For this review, take the finished solid that the model builds, in its own axes (mm). A direction names the side the tool comes from. Round coordinates to 2 decimals unless told otherwise and drop trailing zeros. Write each loop counter-clockwise with the first axis right and the second up, starting at its lowest first coordinate (ties: lowest second). Pieces come first, ordered by that corner, then holes. Notation, with made-up numbers: (10, 10) -> (63, 10) arc R19 cw to (63, 19) -> close; hole circle Ø1 at (-15, 35.5). An arc over 180 degrees is marked (long way). Answer in a Markdown table with one row per item.
from build123d import *

# Parameters (mm, degrees)
SKETCH1_R                       = 13.75
BOSS_EXTRUDE1_DEPTH             = 60
SKETCH5_R                       = 10.75
BOSS_EXTRUDE2_DEPTH             = 14.9
CUT_EXTRUDE1_START              = -20
CUT_EXTRUDE1_DEPTH              = 20
CUT_EXTRUDE2_DEPTH              = 64.072379058
CUT_EXTRUDE2_DEPTH_BACK         = 64.072379058
SKETCH7_R                       = 2.625
BOSS_EXTRUDE3_REACH             = 65.072
SKETCH8_R                       = 2.625
BOSS_EXTRUDE3_DIRECTION_2_REACH = 65.072
SKETCH9_R                       = 12.75
SKETCH9_R_2                     = 2.5
CUT_EXTRUDE3_DEPTH              = 10


with BuildPart() as part:
    # Sketch1 → Boss-Extrude1 (new body)
    with BuildSketch(Plane(origin=(0, 0, 0), x_dir=(1, 0, 0), z_dir=(0, 1, 0))):
        with Locations(Location((0, 0, 0), (0, 0, 270))):
            Circle(SKETCH1_R)
    extrude(amount=BOSS_EXTRUDE1_DEPTH)

    # Sketch5 → Boss-Extrude2 (add)
    with BuildSketch(Plane.XZ):
        with Locations(Location((0, 0, 0), (0, 0, 90))):
            Circle(SKETCH5_R)
        with BuildLine():
            Line((0.75, -9.219544457), (0.75, 9.219544457))
            ThreePointArc((0.75, 9.219544457), (9.25, 0), (0.75, -9.219544457))
        make_face(mode=Mode.SUBTRACT)
        with BuildLine():
            Line((-0.75, 9.219544457), (-0.75, -9.219544457))
            ThreePointArc((-0.75, -9.219544457), (-9.25, 0), (-0.75, 9.219544457))
        make_face(mode=Mode.SUBTRACT)
    extrude(amount=BOSS_EXTRUDE2_DEPTH)

    # Sketch6 → Cut-Extrude1 (cut)
    with BuildSketch(Plane.XZ.offset(CUT_EXTRUDE1_START)):
        with BuildLine():
            Line((-0.75, -9.219544457), (-0.75, 9.219544457))
            ThreePointArc((-0.75, 9.219544457), (-9.25, 0), (-0.75, -9.219544457))
        make_face()
        with BuildLine():
            ThreePointArc((0.75, -9.219544457), (9.25, 0), (0.75, 9.219544457))
            Line((0.75, 9.219544457), (0.75, -9.219544457))
        make_face()
    extrude(amount=CUT_EXTRUDE1_DEPTH, mode=Mode.SUBTRACT)

    # Sketch7 → Cut-Extrude2 (cut, two sides: drawn at the far end of the back side and taken through both)
    with BuildSketch(Plane(origin=(0, 0, 0), x_dir=(0, 0, -1), z_dir=(1, 0, 0)).offset(-CUT_EXTRUDE2_DEPTH_BACK)):
        with Locations((0, -10)):
            Circle(SKETCH7_R)
    extrude(amount=CUT_EXTRUDE2_DEPTH + CUT_EXTRUDE2_DEPTH_BACK, mode=Mode.SUBTRACT)

    # Boss-Extrude3: up to this face of the body (flat: up to its plane)
    boss_extrude3_end = Plane(part.part.faces().sort_by_distance((0.75, 2.986865704, 0))[0])
    # Sketch8 → Boss-Extrude3 (add, up to the picked face)
    with BuildSketch(Plane(origin=(0, 0, 0), x_dir=(0, 0, -1), z_dir=(1, 0, 0)), mode=Mode.PRIVATE) as boss_extrude3_sk1:
        with Locations((0, -10)):
            Circle(SKETCH8_R)
    boss_extrude3_tool1 = split(extrude(boss_extrude3_sk1.sketch, amount=BOSS_EXTRUDE3_REACH, mode=Mode.PRIVATE), bisect_by=boss_extrude3_end, keep=Keep.BOTH, mode=Mode.PRIVATE)
    add(boss_extrude3_tool1.solids().sort_by(Axis((0, -10, 0), (1, 0, 0)))[0])

    # Boss-Extrude3 direction 2: up to this face of the body (flat: up to its plane)
    boss_extrude3_direction_2_end = Plane(part.part.faces().sort_by_distance((-0.75, 2.986865704, 0))[0])
    # Sketch8 → Boss-Extrude3 direction 2 (add, up to the picked face)
    with BuildSketch(Plane(origin=(0, 0, 0), x_dir=(0, 0, -1), z_dir=(1, 0, 0)), mode=Mode.PRIVATE) as boss_extrude3_direction_2_sk1:
        with Locations((0, -10)):
            Circle(SKETCH8_R)
    boss_extrude3_direction_2_tool1 = split(extrude(boss_extrude3_direction_2_sk1.sketch, amount=-BOSS_EXTRUDE3_DIRECTION_2_REACH, mode=Mode.PRIVATE), bisect_by=boss_extrude3_direction_2_end, keep=Keep.BOTH, mode=Mode.PRIVATE)
    add(boss_extrude3_direction_2_tool1.solids().sort_by(Axis((0, -10, 0), (-1, 0, 0)))[0])

    # Sketch9 → Cut-Extrude3 (cut)
    with BuildSketch(Plane(origin=(0, 60, 0), x_dir=(1, 0, 0), z_dir=(0, 1, 0))):
        with Locations(Location((0, 0, 0), (0, 0, 270))):
            Circle(SKETCH9_R)
        with Locations(Location((0, 0, 0), (0, 0, 270))):
            Circle(SKETCH9_R_2, mode=Mode.SUBTRACT)
    extrude(amount=-CUT_EXTRUDE3_DEPTH, mode=Mode.SUBTRACT)


solid = part.part
1) Consider section C-C on y = 14. State the section outline as (x, z) points.
Solved:
| item | result |
|---|---|
| outline | circle Ø27.5 at (0, 0); hole (-0.75, -9.22) -> (-0.75, 9.22) arc R9.25 ccw to start; hole (0.75, -9.22) arc R9.25 ccw to (0.75, 9.22) -> close |
2) Mouldability with a two-part tool opening along Z and no side actions: class faces 1 (the flat face through (-3, 50, 0)), 2 (the cylindrical face through (-3.229, -7.346, 10.254)), 3 (the flat face through (-8.1, 60, 10.1)) as pulls with the +Z half, pulls with the -Z half, needs draft (parallel to the pull), parting line crosses it, or undercut.
Solved:
| item | result |
|---|---|
| face 1 | undercut |
| face 2 | parting line crosses it |
| face 3 | needs draft |
3) Clearance check with flat-ended pins moving along their axes: pin 1 Ø12 at (x, z) = (10.5, 2.5) entering from -Y; pin 2 Ø4 at (x, z) = (-6, 2.5) entering from -Y; pin 3 Ø4 at (y, z) = (-10, 0) entering from -X; pin 4 Ø2 at (x, y) = (4, 38.5) entering from +Z. State where each tip first meets the part, or that it passes through.
Solved:
| item | result |
|---|---|
| pin 1 | y = -14.9 |
| pin 2 | y = 20 |
| pin 3 | x = -0.75 |
| pin 4 | z = 13.42 |
4) Consider section A-A on z = 0. State how many separate pieces and enclosed holes the cut face has, then the cut area to 3 significant figures.
Solved:
| item | result |
|---|---|
| separate pieces | 3 |
| enclosed holes | 0 |
| area | 1,160 mm² |
5) For faces 4 (the flat face through (4, 20, 0)), 5 (the cylindrical face through (-9.827, -11.005, -2.425)), 6 (the cylindrical face through (-12.447, 55.07, -2.764)), list the 3-axis set-ups (+Z, -Z, +X, -X, +Y, -Y) from which the entire face can be reached by the end or side of a thin tool; tool diameter is ignored.
Solved:
| item | result |
|---|---|
| face 4 | -Y |
| face 5 | -X |
| face 6 | +Y |
6) Consider section D-D on z = 11.5. State the section outline as (x, y) points, then the cut area to 3 significant figures.
Solved:
| item | result |
|---|---|
| outline | (-7.54, 0) -> (7.54, 0) -> (7.54, 60) -> (5.51, 60) -> (5.51, 50) -> (-5.51, 50) -> (-5.51, 60) -> (-7.54, 60) -> close |
| area | 794 mm² |
7) Consider section B-B on x = 0. State the section outline as (y, z) points, then the cut area to 3 significant figures.
Solved:
| item | result |
|---|---|
| outline | (-14.9, -10.75) -> (0, -10.75) -> (0, -13.75) -> (60, -13.75) -> (60, -12.75) -> (50, -12.75) -> (50, -2.5) -> (60, -2.5) -> (60, 2.5) -> (50, 2.5) -> (50, 12.75) -> (60, 12.75) -> (60, 13.75) -> (0, 13.75) -> (0, 10.75) -> (-14.9, 10.75) -> close |
| area | 1,770 mm² |
8) For line 1 (X direction, y = 56.25, z = 0); line 2 (X direction, y = -2, z = -6.5); line 3 (Y direction, x = -9.45, z = 0) (3 decimals), list the stretches that pass through material, from the lowest coordinate up. Write a range as [from, to].
Solved:
| item | result |
|---|---|
| line 1 | [-13.75, -12.75], [-2.5, 2.5], [12.75, 13.75] |
| line 2 | [-8.56, -6.58], [-0.75, 0.75], [6.58, 8.56] |
| line 3 | [-14.9, -12.625], [-7.375, 50] |
